Autodesk Fusion 360 part; units mm, degrees
sketch "Sketch1" plane through (0, 0, 0) normal (0, 0, 1) x (1, 0, 0)
  line L0 (28, -35) -> (-28, -35)
  line L1 (-30, -33) -> (-30, 33)
  line L2 (-28, 35) -> (28, 35)
  line L3 (30, 33) -> (30, -33)
  line L4 (30, -35) -> (-30, 35) construction
  line L5 (-30, -35) -> (30, 35) construction
  arc A0 (-28, 35) -> (-30, 33) centre (-28, 33) ccw
  arc A1 (30, 33) -> (28, 35) centre (28, 33) ccw
  arc A2 (28, -35) -> (30, -33) centre (28, -33) ccw
  arc A3 (-30, -33) -> (-28, -35) centre (-28, -33) ccw
  circle A4 centre (-20, -29) radius 3
  line L6 (0, 0) -> (0, -32) construction
  line L7 (0, 0) -> (-27.3192, 0) construction
  circle A5 centre (20, -29) radius 3
  circle A6 centre (-20, 29) radius 3
  circle A7 centre (20, 29) radius 3
  dimension "d1" = 60
  dimension "d2" = 70
  dimension "d3" = 2
  dimension "d4" = 6
  dimension "d5" = 10
  dimension "d6" = 6
extrude "Extrude1" add sketch "Sketch1" along normal blind 3
The listing builds one solid part. Answer for the finished solid, in the listing's coordinates (mm). Give positions to 0.01 mm unless a question says otherwise; leave off trailing zeros. Loops run counter-clockwise (first coordinate to the right, second up) from the corner with the lowest first, then second, coordinate; pieces in that order, holes last. Notation, with made-up numbers: (20.25, -30.5) - (29.25, -30.5) arc R30 ccw to (29.25, 4.5) - close; hole circle Ø2 at (25, 26.25). An arc over 180 degrees is marked (long way). Use one line per item in the form item = value.
1. The mould has two halves that part along Y. Classify faces 1 (the face through (0, -35, 1)), 2 (the face through (17, 29, 1)), 3 (the face through (0, 0, 3)), 4 (the face through (-23, 29, 1)): pulls with the +Y half, pulls with the -Y half, needs draft (parallel to the pull), parting line crosses it, or undercut.
Calculated:
face_1 = pulls with the -Y half
face_2 = undercut
face_3 = needs draft
face_4 = undercut
2. Section A-A on y = 29 is taken. Give the vertices of the cut face in (x, z), then the cut area to 3 significant figures.
Calculated:
outline = (-30, 0) - (-23, 0) - (-23, 3) - (-30, 3) - close; (-17, 0) - (17, 0) - (17, 3) - (-17, 3) - close; (23, 0) - (30, 0) - (30, 3) - (23, 3) - close
area = 144 mm^2
3. Section C-C on x = -20 is taken. Give the vertices of the cut face in (y, z).
Calculated:
outline = (-35, 0) - (-32, 0) - (-32, 3) - (-35, 3) - close; (-26, 0) - (26, 0) - (26, 3) - (-26, 3) - close; (32, 0) - (35, 0) - (35, 3) - (32, 3) - close
4. Find the intervals of material crossed by line 1 along Y through (x, z) = (20, 1.05); line 2 along Y through (x, z) = (18, 0.2), in increasing order. Write a range as [from, to].
Calculated:
line_1 = [-35, -32], [-26, 26], [32, 35]
line_2 = [-35, -31.24], [-26.76, 26.76], [31.24, 35]
5. Section B-B on z = 1.15 is taken. Give the vertices of the cut face in (x, y), then the cut area to 3 significant figures.
Calculated:
outline = (-30, -33) arc R2 ccw to (-28, -35) - (28, -35) arc R2 ccw to (30, -33) - (30, 33) arc R2 ccw to (28, 35) - (-28, 35) arc R2 ccw to (-30, 33) - close; hole circle Ø6 at (-20, -29); hole circle Ø6 at (-20, 29); hole circle Ø6 at (20, -29); hole circle Ø6 at (20, 29)
area = 4,080 mm^2
